CAD build for the part. Positions are in the model's coordinates, mm. Round coordinates to 2 decimals unless told otherwise and drop trailing zeros. Loops run counter-clockwise (first coordinate to the right, second up) from the corner with the lowest first, then second, coordinate; pieces in that order, holes last. Notation, with made-up numbers: (66.25, -31.5) - (124.25, -31.5) arc R23 ccw to (124.25, -7.5) - close; hole circle Ø10 at (41, 66.5). An arc over 180 degrees is marked (long way). One line per question, with ' | ' between items.
```python
from build123d import *

# Parameters (mm, degrees)
SKETCH_1_R          = 10
SKETCH_1_R_2        = 7.5
EXTRUDE_1_DEPTH     = 450
SKETCH_2_R          = 1
CUT_EXTRUDE_2_DEPTH = 20
SKETCH_3_R          = 1
CUT_EXTRUDE_3_DEPTH = 20


with BuildPart() as part:
    # Эскиз1 → Вытянуть1 (new body)
    with BuildSketch(Plane.XY):
        Circle(SKETCH_1_R)
        Circle(SKETCH_1_R_2, mode=Mode.SUBTRACT)
    extrude(amount=EXTRUDE_1_DEPTH)

    # Эскиз2 → Вытянуть2 (cut, symmetric)
    with BuildSketch(Plane(origin=(0, 0, 0), x_dir=(1, 0, 0), z_dir=(0, 1, 0))):
        with Locations(Location((0, -5, 0), (0, 0, 270))):
            Circle(SKETCH_2_R)
    extrude(amount=CUT_EXTRUDE_2_DEPTH, both=True, mode=Mode.SUBTRACT)

    # Эскиз3 → Вытянуть3 (cut, symmetric)
    with BuildSketch(Plane(origin=(0, 0, 0), x_dir=(1, 0, 0), z_dir=(0, 1, 0))):
        with Locations(Location((0, -444, 0), (0, 0, 270))):
            Circle(SKETCH_3_R)
    extrude(amount=CUT_EXTRUDE_3_DEPTH, both=True, mode=Mode.SUBTRACT)


solid = part.part
```
(1) Probe L1, parallel to Z at x = 0, y = 8.2; L2, parallel to Y at x = 1.25, z = 336; L3, parallel to X at y = -1, z = 99. List the from-to ranges inside material, lowest first.
Results found:
L1: z = 0 to 4, 6 to 443, 445 to 450 | L2: y = -9.92 to -7.4, 7.4 to 9.92 | L3: x = -9.95 to -7.43, 7.43 to 9.95
(2) Drop flat-ended pins along their axis: P1, Ø12, axis at y = -6.5, z = 135.5, coming from the -X side; P2, Ø4, axis at y = 6.5, z = 267.5, coming from the +X side; P3, Ø12, axis at x = 3.5, z = 174, coming from the +Y side; P4, Ø1.5, axis at x = 4.5, z = 225.5, coming from the +Y side. Give the stop position or say it passes through.
Results found:
P1: stops at x = -9.99 | P2: stops at x = 8.93 | P3: stops at y = 10 | P4: stops at y = 9.27
(3) Two-plate mould, pull along X, no slides. Class faces 1 (the face through (4, 7, 0)), 2 (the face through (-7.493, 0.33, 221.85)), 3 (the face through (-2.17, -9.76, 221.85)): released by +X, released by -X, zero draft, split by the parting line, or undercut.
Results found:
face 1: zero draft | face 2: undercut | face 3: split by the parting line
(4) Cut at A-A, the plane z = 28. Write the cut outline in (x, y), then the cut area to 3 significant figures.
Results found:
outline: circle Ø20 at (0, 0); hole circle Ø15 at (0, 0) | area: 137 mm²
